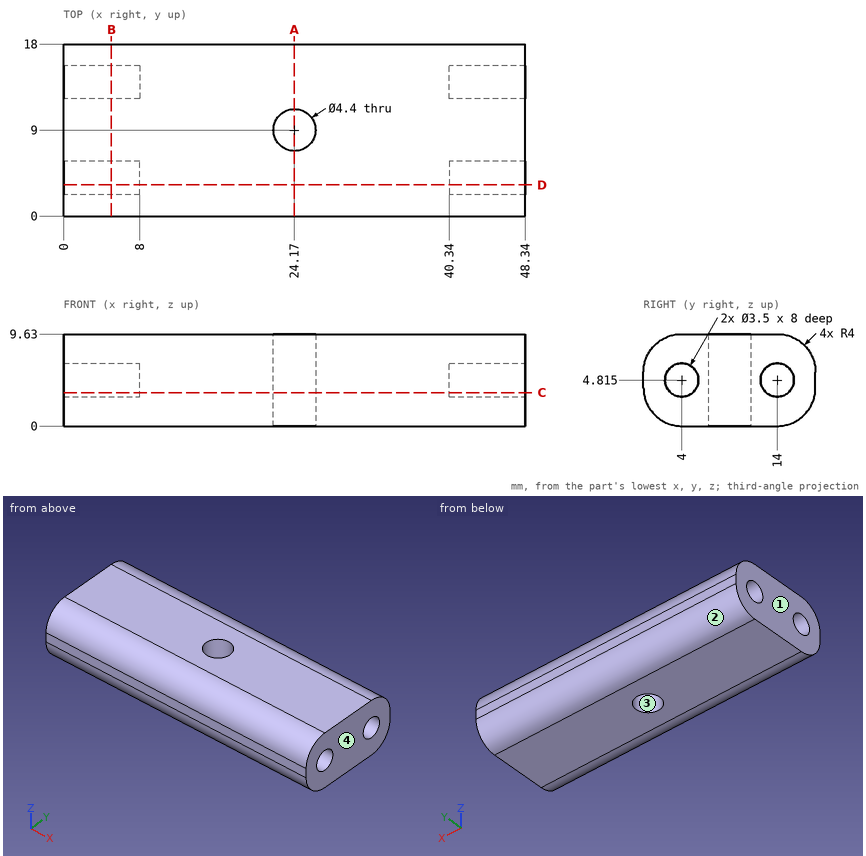
The figure shows three views and two pictorial views of one solid part (mm, origin at its lowest corner). Answer the questions. Round coordinates to 2 decimals unless told otherwise and drop trailing zeros. Write each loop counter-clockwise with the first axis right and the second up, starting at its lowest first coordinate (ties: lowest second). Pieces come first, ordered by that corner, then holes. Notation, with made-up numbers: (-26.75, 64.25) - (18.25, 64.25) arc R20 ccw to (18.25, 103.25) - close; hole circle Ø10 at (-1, 18). An arc over 180 degrees is marked (long way). One line per question, with ' | ' between items. Start each with the question number.
1. For a pull along X with two mould halves and no side action, classify the marked faces 1, 2, 3 and 4 as +X half, -X half, draft (parallel to the pull), parting line (faces both ways), or undercut.
2. Each of these flat-tipped pins is pushed along its axis until it touches: pin 1 (1.8 mm diameter, centred on y = 3.5, z = 5, fed in from +X); pin 2 (1 mm diameter, centred on x = 23, z = 7.5, fed in from +Y); pin 3 (2 mm diameter, centred on y = 14, z = 4.815, fed in from -X); pin 4 (4 mm diameter, centred on x = 24.17, y = 9, fed in from -Z). Where does it stop, or does it pass through?
3. Section D-D (y = 3.25) is taken. Determine the outline of the cut face in (x, z).
4. Section C-C (z = 3.5) is taken. Determine the outline of the cut face in (x, y).
5. Section B-B (x = 5) is taken. Determine the outline of the cut face in (y, z) (3 decimals), and give its area (3 significant figures).
6. Find the intervals of material crossed by probe 1 along Y at (x, z) = (4, 6); probe 2 along Y at (x, z) = (46.5, 3.25); probe 3 along X at (y, z) = (15, 5.25), in increasing order. Write a range as [from, to].
7. Section A-A (x = 24.17) is taken. Determine the outline of the cut face in (y, z), and give its area (3 significant figures).
Filled in:
1) face 1: -X half | face 2: draft | face 3: undercut | face 4: +X half
2) pin 1: x = 40.34 | pin 2: y = 17.76 | pin 3: x = 8 | pin 4: through
3) outline: (0, 0.07) - (48.34, 0.07) - (48.34, 3.23) - (40.34, 3.23) - (40.34, 6.4) - (48.34, 6.4) - (48.34, 9.56) - (0, 9.56) - (0, 6.4) - (8, 6.4) - (8, 3.23) - (0, 3.23) - close
4) outline: (0, 0.03) - (48.34, 0.03) - (48.34, 2.85) - (40.34, 2.85) - (40.34, 5.15) - (48.34, 5.15) - (48.34, 12.85) - (40.34, 12.85) - (40.34, 15.15) - (48.34, 15.15) - (48.34, 17.97) - (0, 17.97) - (0, 15.15) - (8, 15.15) - (8, 12.85) - (0, 12.85) - (0, 5.15) - (8, 5.15) - (8, 2.85) - (0, 2.85) - close; hole circle Ø4.4 at (24.17, 9)
5) outline: (0, 4) arc R4 ccw to (4, 0) - (14, 0) arc R4 ccw to (18, 4) - (18, 5.63) arc R4 ccw to (14, 9.63) - (4, 9.63) arc R4 ccw to (0, 5.63) - close; hole circle Ø3.5 at (4, 4.815); hole circle Ø3.5 at (14, 4.815) | area: 140 mm²
6) probe 1: [0.02, 2.71], [5.29, 12.71], [15.29, 17.98] | probe 2: [0.07, 3.22], [4.78, 13.22], [14.78, 17.93] | probe 3: [8, 40.34]
7) outline: (0, 4) arc R4 ccw to (4, 0) - (6.8, 0) - (6.8, 9.63) - (4, 9.63) arc R4 ccw to (0, 5.63) - close; (11.2, 0) - (14, 0) arc R4 ccw to (18, 4) - (18, 5.63) arc R4 ccw to (14, 9.63) - (11.2, 9.63) - close | area: 117 mm²
